from build123d import *

# Parameters (mm, degrees)
F1_DEPTH = 81.026
F2_R     = 78.74
F3_DEPTH = 233.68
F4_R     = 124.3645263244
F5_DEPTH = 2.286
F7_R     = 5.08


# Not quite as in the source:
# - a fillet or chamfer that OpenCascade refuses, or shapes differently, is made with other operations: its cross-section is extruded or revolved along the edge and cut away or added


with BuildPart() as f1:
    # F0 (on Top) → F1 (new body)
    with BuildSketch(Plane.XY):
        Polygon((46.9164714903, -142.236754682), (146.6388786516, -30.4875211745), (99.7224071613, 111.7492335075), (-46.9164714903, 142.236754682), (-146.6388786516, 30.4875211745), (-99.7224071613, -111.7492335075), align=None)
    extrude(amount=F1_DEPTH)

    # F2 (on face) → F3 (join)
    with BuildSketch(Plane.XY.offset(81.026)):
        Circle(F2_R)
    extrude(amount=F3_DEPTH)

    # F4 (on face) → F5 (join)
    with BuildSketch(Plane(origin=(0, 0, 0), x_dir=(1, 0, 0), z_dir=(0, 0, -1))):
        Circle(F4_R)
    extrude(amount=F5_DEPTH)

    # F6: fillet of radius 10.6614809392 on 1 edges, made by hand

    # F6_s1 → F6_t2 (revolve, cut)
    with BuildSketch(Plane.XZ):
        with BuildLine():
            ThreePointArc((124.3645263244, 0), (121.2585269877, -1.6983020197), (117.767671403, -2.286))
            Line((117.767671403, -2.286), (124.3645263244, -2.286))
            Line((124.3645263244, -2.286), (124.3645263244, 0))
        make_face()
    revolve(axis=Axis((0, 0, -2.286), (0, 0, -1)), mode=Mode.SUBTRACT)

    # F7
    f7_edges = [f1.edges().sort_by_distance(p)[0] for p in [
        (-124.364526, 0, 0),
    ]]
    fillet(f7_edges, radius=F7_R)


solid = f1.part
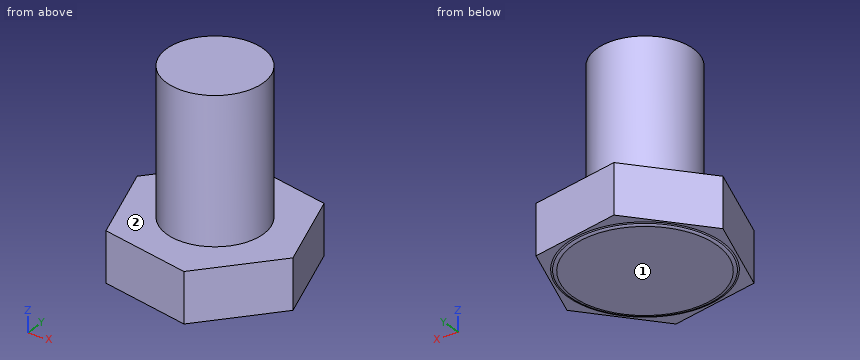
Work out the finished part from the listing and answer in its coordinate system (mm). Face numbers are marked on the shaded views. A direction names the side the tool comes from. Round coordinates to 2 decimals unless told otherwise and drop trailing zeros. Write each loop counter-clockwise with the first axis right and the second up, starting at its lowest first coordinate (ties: lowest second). Pieces come first, ordered by that corner, then holes.
1) Straight lines are drawn through the part: line 1 (X direction, y = -1, z = 94); line 2 (Z direction, x = 59, y = 102.5); line 3 (Y direction, x = 3.5, z = 186.5). For each, find the intervals that lie inside material, in ascending order.
2) A cutting plane is placed at B-B (z = 233). Give the vertices of the cut face in (x, y).
3) A tool of negligible diameter and unlimited length cuts with its end or side. For the marked faces 1 and 2, from which of +Z, -Z, +X, -X, +Y, -Y can it reach the whole face along a straight path? Write none if from no direction.
4) A cutting plane is placed at A-A (z = 27). Give the vertices of the cut face in (x, y).
5) Given pin 1 Ø2 at (x, z) = (-8, 236) entering from +Y; pin 2 Ø2 at (y, z) = (0.5, 93) entering from +X; pin 3 Ø1 at (x, y) = (-95, -106) entering from -Z; pin 4 Ø10 at (x, y) = (-26, -74.5) entering from +Z, each flat-ended and moving along its own axis, determine where each tip first touches the part or whether it passes through.
Completed:
1. line 1: x = -78.73 to 78.73
1. line 2: z = -2.27 to 81.03
1. line 3: y = -78.66 to 78.66
2. outline: circle Ø157.48 at (0, 0)
3. face 1: -Z, +X, -X, +Y, -Y
3. face 2: +Z
4. outline: (-146.64, 30.49) - (-99.72, -111.75) - (46.92, -142.24) - (146.64, -30.49) - (99.72, 111.75) - (-46.92, 142.24) - close
5. pin 1: stops at y = 78.43
5. pin 2: stops at x = 78.74
5. pin 3: stops at z = 0
5. pin 4: stops at z = 314.71
